Can you work these out from the model? Positions are in its coordinate system, mm. Face numbers are marked on the shaded views. A direction names the side the tool comes from. Give positions to 0.01 mm unless a question says otherwise; leave off trailing zeros. Loops run counter-clockwise (first coordinate to the right, second up) from the corner with the lowest first, then second, coordinate; pieces in that order, holes last. Notation, with made-up numbers: (23, 87.25) - (41, 87.25) arc R33 cw to (41, 115.25) - close; hole circle Ø11 at (-40, 77.5). An arc over 180 degrees is marked (long way). Answer in a Markdown table with one row per item.
Autodesk Inventor part; units mm, degrees
ref_plane "Work Plane1" through (0, 0, -15) normal (0, 0, 1) x (1, 0, 0)
ref_plane "YZ Plane" through (0, 0, 0) normal (1, 0, 0) x (0, 1, 0)
ref_plane "XZ Plane" through (0, 0, 0) normal (0, 1, 0) x (-1, 0, 0)
sketch "Sketch1" plane through (0, 0, 0) normal (0, 0, 1) x (1, 0, 0)
  line L0 (0, 0) -> (25, 0)
  line L1 (25, 0) -> (25, 40)
  line L2 (25, 40) -> (0, 40)
  line L3 (0, 40) -> (0, 0)
  dimension "d1" = 25
  dimension "d2" = 40
  dimension "d3" = 25
extrude "Extrusion1" add sketch "Sketch1" against normal blind 30
sketch "Sketch2" plane through (25, 0, 0) normal (1, 0, 0) x (0, 0, -1)
  line L0 (0, 0) -> (30, 0)
  circle A0 centre (15, 6.56) radius 2.46
extrude "Extrusion2" cut sketch "Sketch2" against normal blind 30
sketch "Sketch3" plane through (0, 0, 0) normal (-1, 0, 0) x (0, 0, 1)
  line L0 (0, 0) -> (-30, 0)
  line L1 (-25.05, 0) -> (-4.95, 0)
  line L2 (-4.95, 0) -> (-4.95, 33.12)
  line L3 (-4.95, 33.12) -> (-25.05, 33.12)
  line L4 (-25.05, 33.12) -> (-25.05, 0)
  dimension "d11" = 20.1
extrude "Extrusion3" cut sketch "Sketch3" against normal blind 20
sketch "Sketch4" plane through (0, 0, 0) normal (0, -1, 0) x (1, 0, 0)
  line L0 (20, -4.95) -> (20, -25.05)
  line L1 (20, -15) -> (25, -15)
  line L2 (25, 0) -> (25, -30)
  line L3 (20, -8.025) -> (25, -8.025)
  line L4 (25, -8.025) -> (25, -21.975)
  line L5 (25, -21.975) -> (20, -21.975)
  line L6 (20, -21.975) -> (20, -8.025)
  line L7 (20, -8.025) -> (25, -21.975) construction
  line L8 (25, -8.025) -> (20, -21.975) construction
  line L9 (25, -12.54) -> (25, -17.46)
  point P0 (0, 0)
  point P1 (22.5, -15)
  dimension "d14" = 13.95
extrude "Extrusion4" add sketch "Sketch4" along normal blind 15
sketch "Sketch5" plane through (20, 0, 0) normal (-1, 0, 0) x (0, 0, 1)
  circle A0 centre (-15, 6.56) radius 2.46
  circle A1 centre (-15, 6.56) radius 4.7025
  circle A2 centre (-15, 6.56) radius 2.46
  circle A3 centre (-15, 6.56) radius 2.46
  point P0 (0, 0)
  dimension "d17" = 9.405
extrude "Extrusion5" cut sketch "Sketch5" against normal blind 2.1
sketch "Sketch6" plane through (25, 0, 0) normal (1, 0, 0) x (0, 0, -1)
  circle A0 centre (15, 6.56) radius 4.7025
  line L0 (15, 6.56) -> (15, 23.56)
  circle A1 centre (15, 23.56) radius 2.46
  point P0 (0, 0)
  dimension "d20" = 17
  dimension "d21" = 4.92
extrude "Extrusion6" cut sketch "Sketch6" against normal blind 10 contours A1
sketch "Sketch7" plane through (20, 0, 0) normal (-1, 0, 0) x (0, 0, 1)
  circle A0 centre (-15, 23.56) radius 2.46
  circle A1 centre (-15, 23.56) radius 4.7025
  point P0 (0, 0)
  dimension "d24" = 9.405
extrude "Extrusion7" cut sketch "Sketch7" against normal blind 2.1
sketch "Sketch9" plane through (25, 0, 0) normal (1, 0, 0) x (0, 0, -1)
  circle A0 centre (15, 6.56) radius 2.46
  circle A1 centre (15, 6.56) radius 2.46
  circle A2 centre (15, 23.56) radius 2.46
  circle A3 centre (15, 23.56) radius 2.46
  line L0 (30, 40) -> (30, 0)
  line L1 (30, 0) -> (30, 40)
  line L2 (30, 40) -> (0, 40)
  line L3 (0, 40) -> (0, 0)
  line L4 (0, 0) -> (8.025, 0)
  line L5 (21.975, 0) -> (21.975, -15)
  line L6 (21.975, -15) -> (8.025, -15)
  line L7 (8.025, -15) -> (8.025, 0)
  line L8 (0, 0) -> (8.025, 0)
  line L9 (21.975, 0) -> (30, 0)
extrude "Extrusion8" add sketch "Sketch9" along normal blind 5
sketch "Sketch10" plane through (0, 40, 0) normal (0, 1, 0) x (1, 0, 0)
  line L0 (0, 30) -> (30, 30)
  line L1 (30, 0) -> (0, 0)
  line L2 (0, 30) -> (30, 30)
  line L3 (30, 30) -> (30, 0)
  line L4 (30, 0) -> (0, 0)
  line L5 (0, 0) -> (0, 30)
extrude "Extrusion9" add sketch "Sketch10" along normal blind 30
sketch "Sketch12" plane through (30, 0, 0) normal (1, 0, 0) x (0, 0, -1)
  circle A0 centre (15, 6.56) radius 2.46
  line L0 (15, 6.56) -> (15, 15.06)
  circle A1 centre (15, 15.06) radius 2.525
  point P0 (0, 0)
  dimension "d31" = 8.5
  dimension "d33" = 5.05
extrude "Extrusion10" cut sketch "Sketch12" against normal blind 30 contours A1
sketch "Sketch15" plane through (0, 0, -25.05) normal (-1, 0, 0) x (0, 0, 1)
  line L0 (0, 33.12) -> (20.1, 33.12)
  line L1 (20.1, 33.12) -> (20.1, 0)
  line L2 (0, 33.12) -> (20.1, 33.12)
  line L3 (20.1, 33.12) -> (20.1, 31.1)
  line L4 (20.1, 31.1) -> (0, 31.1)
  line L5 (0, 31.1) -> (0, 33.12)
  point P0 (25.05, 0)
  dimension "d57" = 2.02
extrude "Extrusion13" add sketch "Sketch15" against normal blind 20
sketch "Sketch17" plane through (0, 0, 0) normal (0, 0, 1) x (1, 0, 0)
  line L0 (0, 70) -> (30, 70)
  line L1 (30, 70) -> (50.0622, 90.0622)
  line L2 (30, 70) -> (80, 70) construction
  line L3 (11.9522, 97.2454) -> (0, 85.2932)
  line L4 (0, 70) -> (0, 85.2932)
  line L5 (0, 70) -> (0, 0)
  line L6 (0, 70) -> (30, 70)
  line L7 (10.923, 112.2849) -> (0, 120.567)
  line L8 (50.0622, 105.3553) -> (50.0622, 120.567)
  line L9 (50.0622, 105.3553) -> (50.0622, 90.0622)
  arc A0 (11.9522, 97.2454) -> (10.923, 112.2849) centre (4.8811, 104.3165) ccw
  line L10 (0, 152.567) -> (30, 152.567)
  line L11 (30, 152.567) -> (50.0622, 120.567)
  line L12 (5, 150.567) -> (0, 152.567)
  line L13 (5, 122.567) -> (0, 120.567)
  line L14 (5, 122.567) -> (10, 136.567)
  line L15 (10, 136.567) -> (5, 150.567)
  dimension "d61" = 45
  dimension "d62" = 32.0271
  dimension "d72" = 10
extrude "Extrusion14" add sketch "Sketch17" against normal blind 30
sketch "Sketch22" plane through (0, 0, 0) normal (0, 0, 1) x (1, 0, 0)
  line L0 (30, 0) -> (30, 70)
  line L1 (50.0622, 90.0622) -> (30, 70)
  line L2 (30, 70) -> (50.0622, 90.0622)
  line L3 (50.0622, 120.567) -> (50.0622, 90.0622)
  line L4 (50.0622, 90.0622) -> (50.0622, 120.567)
  line L5 (30, 152.567) -> (50.0622, 120.567)
  line L6 (50.0622, 120.567) -> (30, 152.567)
  line L7 (0, 152.567) -> (30, 152.567)
  line L8 (30, 152.567) -> (0, 152.567)
  line L9 (5, 150.567) -> (0, 152.567)
  line L10 (0, 152.567) -> (5, 150.567)
  line L11 (5, 150.567) -> (10, 136.567)
  line L12 (5, 150.567) -> (10, 136.567)
  line L13 (10, 136.567) -> (5, 122.567)
  line L14 (10, 136.567) -> (5, 122.567)
  line L15 (5, 122.567) -> (0, 120.567)
  line L16 (5, 122.567) -> (0, 120.567)
  line L17 (0, 120.567) -> (10.923, 112.2849)
  line L18 (0, 120.567) -> (10.923, 112.2849)
  line L19 (0, 85.2932) -> (11.9522, 97.2454)
  line L20 (11.9522, 97.2454) -> (0, 85.2932)
  line L21 (0, 85.2932) -> (0, 55.2932)
  line L22 (0, 0) -> (0, 85.2932)
  line L23 (0, 55.2932) -> (30, 55.2932)
  line L24 (30, 55.2932) -> (30, 70)
  arc A0 (11.9522, 97.2454) -> (10.923, 112.2849) centre (4.8811, 104.3165) ccw
  dimension "d92" = 30
extrude "Extrusion15" add sketch "Sketch22" along normal blind 30
ref_plane "Work Plane1" through (0, 0, -15) normal (0, 0, 1) x (1, 0, 0)
mirror "Mirror1" about plane through (0, 0, -15) normal (0, 0, 1) of "Extrusion15"
properties part number "rec_c_28mm_x_90mm"
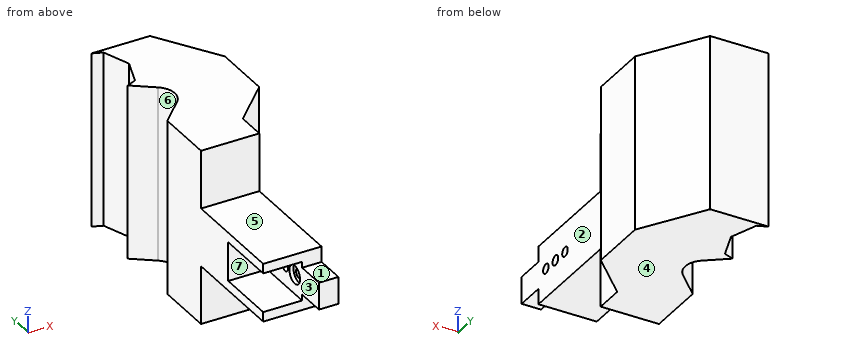
Q1. Imagine slicing it at A-A, the plane y = 15.06. Write out the boundary of the cut face in (x, z) (3 decimals), and give its area (4 significant figures).
Checked values:
| item | result |
|---|---|
| outline | (0, -30) - (30, -30) - (30, -17.525) - (20, -17.525) - (20, -25.05) - (0, -25.05) - close; (0, -4.95) - (20, -4.95) - (20, -12.475) - (30, -12.475) - (30, 0) - (0, 0) - close |
| area | 447.5 mm² |
Q2. On a 3-axis mill with a long thin cutter (end or side, diameter ignored), from which of +Z, -Z, +X, -X, +Y, -Y can I reach the whole of each face in a straight line? I mean the marked faces 1, 2 and 3. Say none if no direction works.
Checked values:
| item | result |
|---|---|
| face 1 | +Z, +X, -X, -Y |
| face 2 | +Z, -Z, +X, -Y |
| face 3 | -X, -Y |
Q3. If I drill on line 1 (Y direction, x = 21, z = -15) (1 decimal); line 2 (Y direction, x = 27, z = -15) (3 decimals); line 3 (Z direction, x = 24.5, y = 6.56), over which ranges is the centre line in solid material (lowest first)? Write a range as [from, to].
Checked values:
| item | result |
|---|---|
| line 1 | y = [-15, 1.9], [11.3, 12.5], [17.6, 18.9], [28.3, 152.6] |
| line 2 | y = [-15, 4.1], [9.02, 12.535], [17.585, 21.1], [26.02, 152.567] |
| line 3 | z = [-30, -17.46], [-12.54, 0] |
Q4. Imagine slicing it at C-C, the plane z = 16.5. Write out the boundary of the cut face in (x, y), and give its area (3 significant figures).
Checked values:
| item | result |
|---|---|
| outline | (0, 55.29) - (30, 55.29) - (30, 70) - (50.06, 90.06) - (50.06, 120.57) - (30, 152.57) - (0, 152.57) - (5, 150.57) - (10, 136.57) - (5, 122.57) - (0, 120.57) - (10.92, 112.28) arc R10 cw to (11.95, 97.25) - (0, 85.29) - close |
| area | 3,510 mm² |
Q5. If we mould it in two halves opening along Z, with no side actions, what happens to the marked faces 4, 5, 6 and 7? For each: released by +Z, released by -Z, zero draft, split by the parting line, or undercut.
Checked values:
| item | result |
|---|---|
| face 4 | released by -Z |
| face 5 | released by +Z |
| face 6 | zero draft |
| face 7 | undercut |
Q6. For pin 1 (10 mm diameter, centred on y = 28.5, z = -7, fed in from +X); pin 2 (6 mm diameter, centred on y = 135.5, z = -41.5, fed in from -X); pin 3 (7.5 mm diameter, centred on y = 8.5, z = -13.5, fed in from -X); pin 4 (3 mm diameter, centred on y = 6.56, z = -15, fed in from +X) (3 decimals), each with a flat end and sliding along its axis, tell me the tip position at first contact or that it passes through.
Checked values:
| item | result |
|---|---|
| pin 1 | stops at x = 30 |
| pin 2 | stops at x = 8.55 |
| pin 3 | stops at x = 20 |
| pin 4 | passes through |
Q7. Imagine slicing it at B-B, the plane x = 17. Write out the boundary of the cut face in (y, z), and give its area (3 significant figures).
Checked values:
| item | result |
|---|---|
| outline | (0, -30) - (55.29, -30) - (55.29, -60) - (152.57, -60) - (152.57, 30) - (55.29, 30) - (55.29, 0) - (0, 0) - (0, -4.95) - (31.1, -4.95) - (31.1, -25.05) - (0, -25.05) - close |
| area | 9,790 mm² |
Q8. Imagine slicing it at D-D, the plane z = -15. Count the separate pieces of the cut face and the enclosed holes in it, and give its area (3 significant figures).
Checked values:
| item | result |
|---|---|
| separate pieces | 4 |
| enclosed holes | 0 |
| area | 4,530 mm² |
